Part model, mm, in its own coordinate system. Coordinates: 2 decimals unless noted, no trailing zeros. Order: outer loops, then holes, each group sorted by start corner. A loop starts at its lowest first (then second) coordinate and runs counter-clockwise, first axis right, second up.
from build123d import *

# Parameters (mm, degrees)
F0_W     = 5
F0_H     = 10
F1_DEPTH = 11.25
F2_R     = 2.25
F3_DEPTH = 5.001
F4_R     = 1


with BuildPart() as f1:
    # F0 (on Right) → F1 (new body, symmetric)
    with BuildSketch(Plane.YZ):
        with Locations((2.5, 0)):
            Rectangle(F0_W, F0_H)
    extrude(amount=F1_DEPTH, both=True)

    # F2 (on face) → F3 (cut, through all)
    with BuildSketch(Plane.XZ):
        Circle(F2_R)
    extrude(amount=-F3_DEPTH, mode=Mode.SUBTRACT)

    # F4
    f4_edges = [f1.edges().sort_by_distance(p)[0] for p in [
        (0, 0, 5),
        (0, 0, -5),
        (0, 5, 5),
        (0, 5, -5),
    ]]
    fillet(f4_edges, radius=F4_R)


solid = f1.part
Q1. Wall check: line 1 along Z through (x, y) = (0, 2); line 2 along X through (y, z) = (2.6, 1.25); line 3 along Z through (x, y) = (-1, 1.65). Give the ranges that are in metal, low to high.
Results list:
line 1: z = -5 to -2.25, 2.25 to 5
line 2: x = -11.25 to -1.87, 1.87 to 11.25
line 3: z = -5 to -2.02, 2.02 to 5
Q2. Cut at B-B on y = 1.45. Write the cut outline in (x, z), and give its area (3 significant figures).
Results list:
outline: (-11.25, -5) - (11.25, -5) - (11.25, 5) - (-11.25, 5) - close; hole circle Ø4.5 at (0, 0)
area: 209 mm2
Q3. Cut at C-C on z = 0. Write the cut outline in (x, y), and give its area (3 significant figures).
Results list:
outline: (-11.25, 0) - (-2.25, 0) - (-2.25, 5) - (-11.25, 5) - close; (2.25, 0) - (11.25, 0) - (11.25, 5) - (2.25, 5) - close
area: 90.0 mm2
Q4. Cut at D-D on x = -8. Write the cut outline in (y, z).
Results list:
outline: (0, -4) arc R1 ccw to (1, -5) - (4, -5) arc R1 ccw to (5, -4) - (5, 4) arc R1 ccw to (4, 5) - (1, 5) arc R1 ccw to (0, 4) - close
Q5. Cut at A-A on x = 0. Write the cut outline in (y, z), and give its area (3 significant figures).
Results list:
outline: (0, -4) arc R1 ccw to (1, -5) - (4, -5) arc R1 ccw to (5, -4) - (5, -2.25) - (0, -2.25) - close; (0, 2.25) - (5, 2.25) - (5, 4) arc R1 ccw to (4, 5) - (1, 5) arc R1 ccw to (0, 4) - close
area: 26.6 mm2
Q6. Mould opens along X. For faces 1 (the face through (-0.158, 4.699, 4.715)), 2 (the face through (-0.29, 2.46, 2.23)), 3 (the face through (-11.25, 2, 0)), 4 (the face through (11.25, 2, 0)) say: pulls with the +X half, pulls with the -X half, needs draft (parallel to the pull), parting line crosses it, or undercut.
Results list:
face 1: needs draft
face 2: undercut
face 3: pulls with the -X half
face 4: pulls with the +X half
